Answer from the drawing. Dimensions are ordinates in mm from the lowest x, y and z of the part. Round coordinates to 2 decimals unless told otherwise and drop trailing zeros. Loops run counter-clockwise (first coordinate to the right, second up) from the corner with the lowest first, then second, coordinate; pieces in that order, holes last. Notation, with made-up numbers: M 84,42.25 L 94,42.25 A21 ccw 94,77.25 Z; hole C -40,81.5 d5. An arc over 180 degrees is marked long. Write each question's results on one line, items separated by ' | '.
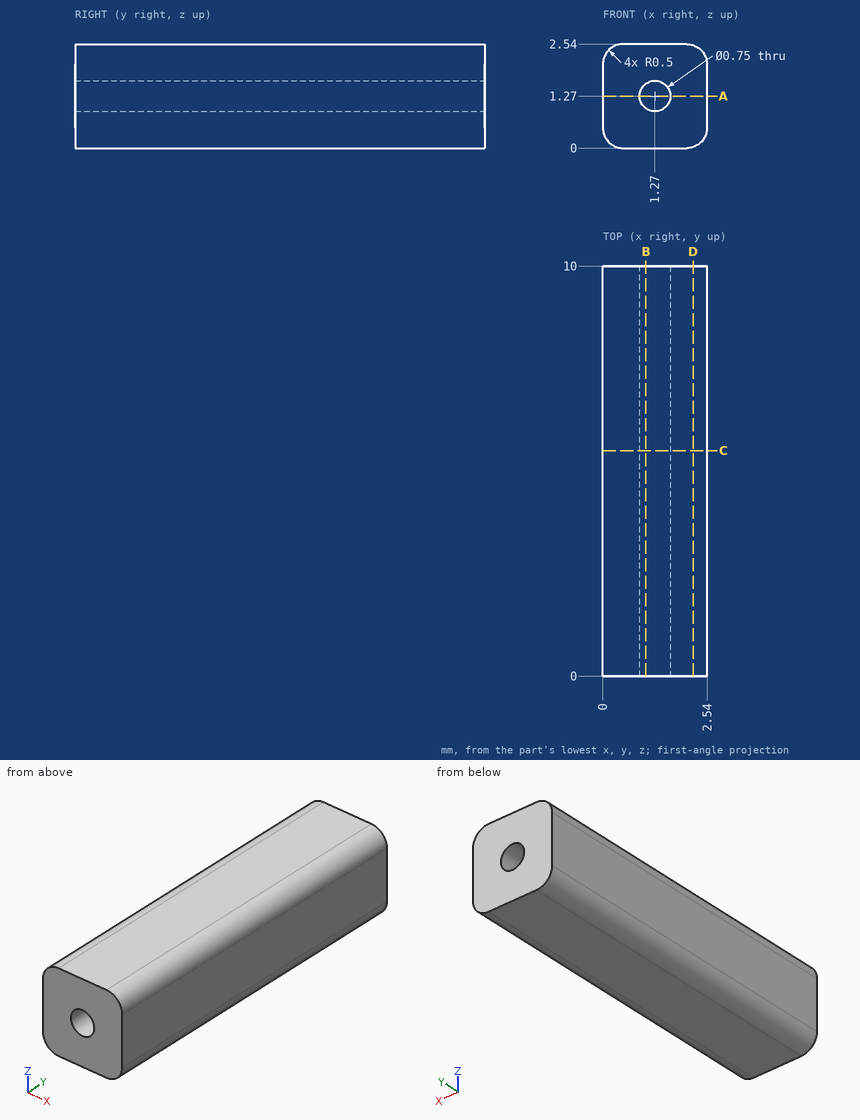
1. Find the intervals of material crossed by L1, parallel to Z at x = 1.27, y = 5.5 (3 decimals); L2, parallel to X at y = 5.75, z = 1.5, in increasing order.
Completed:
L1: z = 0 to 0.895, 1.645 to 2.54 | L2: x = 0 to 0.97, 1.57 to 2.54
2. Find section B-B, the plane x = 1.05. Give the vertices of the cut face in (y, z).
Completed:
outline: M 0,0 L 10,0 L 10,0.97 L 0,0.97 Z; M 0,1.57 L 10,1.57 L 10,2.54 L 0,2.54 Z
3. Find section D-D, the plane x = 2.2. Give the vertices of the cut face in (y, z), then the cut area to 3 significant figures.
Completed:
outline: M 0,0.03 L 10,0.03 L 10,2.51 L 0,2.51 Z | area: 24.9 mm2
4. Find section C-C, the plane y = 5.5. Give the vertices of the cut face in (x, z) (3 decimals), then the cut area to 3 significant figures.
Completed:
outline: M 0,0.5 A0.5 ccw 0.5,0 L 2.04,0 A0.5 ccw 2.54,0.5 L 2.54,2.04 A0.5 ccw 2.04,2.54 L 0.5,2.54 A0.5 ccw 0,2.04 Z; hole C 1.27,1.27 d0.75 | area: 5.80 mm2
5. Find section A-A, the plane z = 1.27. Give the vertices of the cut face in (x, y) (3 decimals).
Completed:
outline: M 0,0 L 0.895,0 L 0.895,10 L 0,10 Z; M 1.645,0 L 2.54,0 L 2.54,10 L 1.645,10 Z
